For this review, use the dimensioned drawing (mm, ordinates from the lowest corner) and the shaded views. Give positions to 0.01 mm unless a question says otherwise; leave off trailing zeros. Order: outer loops, then holes, each group sorted by start corner. A loop starts at its lowest first (then second) coordinate and runs counter-clockwise, first axis right, second up. Notation, with made-up numbers: (77.25, 81.5) - (96.25, 81.5) arc R22 cw to (96.25, 117.5) - close; hole circle Ø11 at (7, -35). An arc over 180 degrees is marked (long way). Use a Markdown table: item, result. Add a question column.
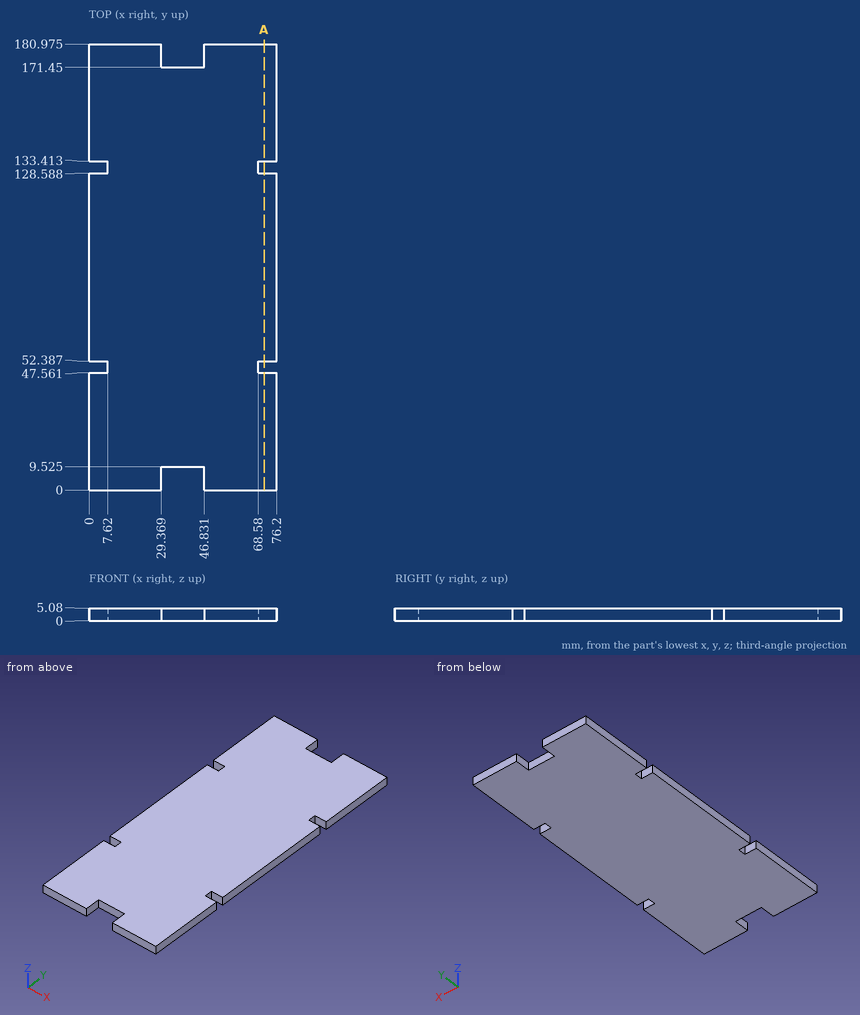
Q1. We need section A-A (x = 71). Write out the cut boundary in (y, z) (1 decimal).
Q2. Wall thickness on probe 1 along Y at (x, z) = (5.5, 0.6) (1 decimal); probe 2 along X at (y, z) = (171.5, 3.2): over which ranges is each line inside the solid? List them lowest first.
Q3. Clearance check with flat-ended pins moving along their axes: P1, Ø2, axis at x = 40, z = 1, coming from the -Y side (1 decimal); P2, Ø1.4, axis at y = 132, z = 3, coming from the -X side. State where each tip first meets the part, or that it passes through.
Here are the results:
| question | item | result |
|---|---|---|
| 1 | outline | (0, 0) - (47.6, 0) - (47.6, 5.1) - (0, 5.1) - close; (52.4, 0) - (128.6, 0) - (128.6, 5.1) - (52.4, 5.1) - close; (133.4, 0) - (181, 0) - (181, 5.1) - (133.4, 5.1) - close |
| 2 | probe 1 | 0 to 47.6, 52.4 to 128.6, 133.4 to 181 |
| 2 | probe 2 | 0 to 29.37, 46.83 to 76.2 |
| 3 | P1 | y = 9.5 |
| 3 | P2 | x = 7.62 |
